Read the model definition and answer for the solid it produces. Units are mm, in the model's axes. A direction names the side the tool comes from. Round coordinates to 2 decimals unless told otherwise and drop trailing zeros. Loops run counter-clockwise (first coordinate to the right, second up) from the corner with the lowest first, then second, coordinate; pieces in that order, holes last. Notation, with made-up numbers: (34.25, -33.75) - (59.25, -33.75) arc R27 ccw to (59.25, -17.75) - close; hole circle Ø2 at (-37.75, -35). An arc over 180 degrees is marked (long way). Use one line per item in the form item = value. Start each with the question number.
Autodesk Inventor part; units mm, degrees
ref_plane "YZ Plane" through (0, 0, 0) normal (1, 0, 0) x (0, 1, 0)
ref_plane "XY Plane" through (0, 0, 0) normal (0, 0, 1) x (1, 0, 0)
sketch "Sketch1" plane through (0, 0, 0) normal (0, 1, 0) x (-1, 0, 0)
  line L0 (0, 4.5) -> (0.254, 4.5)
  line L1 (0.254, -4.5) -> (0, -4.5)
  line L2 (6.35, 4.5) -> (6.35, -4.5)
  line L3 (6.35, 7.548) -> (6.35, 4.5)
  line L4 (6.35, -7.548) -> (6.35, -4.5)
  line L5 (0.254, 4.5) -> (6.35, 7.548)
  line L6 (0.254, -4.5) -> (6.35, -7.548)
  line L7 (0, 4.5) -> (0, -4.5)
  line L8 (0, -20.9) -> (0.254, -20.9)
  line L9 (0.254, -29.9) -> (0, -29.9)
  line L10 (6.35, -20.9) -> (6.35, -29.9)
  line L11 (6.35, -17.852) -> (6.35, -20.9)
  line L12 (6.35, -32.948) -> (6.35, -29.9)
  line L13 (0.254, -20.9) -> (6.35, -17.852)
  line L14 (0.254, -29.9) -> (6.35, -32.948)
  line L15 (0, -20.9) -> (0, -29.9)
  line L16 (0, -46.3) -> (0.254, -46.3)
  line L17 (0.254, -55.3) -> (0, -55.3)
  line L18 (6.35, -46.3) -> (6.35, -55.3)
  line L19 (6.35, -43.252) -> (6.35, -46.3)
  line L20 (6.35, -58.348) -> (6.35, -55.3)
  line L21 (0.254, -46.3) -> (6.35, -43.252)
  line L22 (0.254, -55.3) -> (6.35, -58.348)
  line L23 (0, -46.3) -> (0, -55.3)
  line L24 (0, -71.7) -> (0.254, -71.7)
  line L25 (0.254, -80.7) -> (0, -80.7)
  line L26 (6.35, -71.7) -> (6.35, -80.7)
  line L27 (6.35, -68.652) -> (6.35, -71.7)
  line L28 (6.35, -83.748) -> (6.35, -80.7)
  line L29 (0.254, -71.7) -> (6.35, -68.652)
  line L30 (0.254, -80.7) -> (6.35, -83.748)
  line L31 (0, -71.7) -> (0, -80.7)
  point P0 (0, 0)
  dimension "d16" = 6.096
  dimension "d25" = 9
  dimension "d26" = 3.048
  dimension "d27" = 3.048
  dimension "d28" = 0.254
  dimension "d29" = 0.254
  dimension "d33" = 25.4
extrude "Shape" add sketch "Sketch1" along normal blind 19.05 contours L0 L5 L3 L2 L4 L6 L1 L7 | L8 L13 L11 L10 L12 L14 L9 L15 | L16 L21 L19 L18 L20 L22 L17 L23
sketch "Sketch4" plane through (0, 0, 0) normal (0, -1, 0) x (1, 0, 0)
  line L0 (0, -55.3) -> (-0.254, -55.3) construction
  line L1 (0, -46.3) -> (0, -55.3) construction
  line L2 (-6.35, -43.252) -> (-0.254, -46.3) construction
  line L3 (-6.35, -58.348) -> (-6.35, -43.252) construction
  line L4 (-0.254, -55.3) -> (-6.35, -58.348) construction
  line L5 (-0.254, -46.3) -> (0, -46.3) construction
  line L6 (0, -84.4) -> (-0.254, -84.4)
  line L7 (-0.254, -84.4) -> (-6.35, -81.352)
  line L8 (-6.35, -96.448) -> (-6.35, -81.352)
  line L9 (-0.254, -55.3) -> (-6.35, -58.348)
  line L10 (-0.254, -93.4) -> (-6.35, -96.448)
  line L11 (0, -93.4) -> (-0.254, -93.4)
  line L12 (0, -93.4) -> (0, -84.4)
  line L13 (-0.254, -46.3) -> (0, -46.3)
  line L14 (0, -46.3) -> (0, -55.3)
  point P0 (0, 0)
  dimension "d81" = 38.1
extrude "Extrusion4" add sketch "Sketch4" against normal blind 100.2792
sketch "Sketch5" plane through (0, 0, -84.4) normal (1, 0, 0) x (0, 0, -1)
  line L0 (12.048, 0) -> (12.048, 100.2792) construction
  line L1 (0, 100.2792) -> (9, 100.2792) construction
  line L2 (-91.948, 0) -> (-91.948, 19.05) construction
  line L3 (-76.852, 0) -> (-91.948, 0)
  line L4 (12.048, 0) -> (9, 0)
  line L5 (-91.948, 0) -> (12.048, 0)
  line L6 (9, 100.2792) -> (12.048, 100.2792)
  line L7 (12.048, 0) -> (12.048, 100.2792)
  line L8 (12.048, 100.2792) -> (-13.352, 100.2792)
  line L9 (-13.352, 100.2792) -> (-13.352, 19.05)
  line L10 (-29.1, 19.05) -> (-26.052, 19.05)
  line L11 (-76.852, 19.05) -> (-91.948, 19.05)
  line L12 (-13.352, 19.05) -> (-91.948, 19.05)
  line L13 (-91.948, 19.05) -> (-91.948, 0)
  point P0 (-84.4, 0)
  point P1 (-91.948, 100.2792)
  point P2 (9, 0)
  dimension "d46" = 25.4
extrude "Extrusion5" add sketch "Sketch5" along normal blind 1.27
sketch "Sketch6" plane through (-6.35, 0, -96.448) normal (-1, 0, 0) x (0, 0, 1)
  line L0 (0, 100.2792) -> (15.096, 100.2792)
  line L1 (7.548, 100.2792) -> (7.548, 0) construction
  line L2 (103.996, 0) -> (0, 0)
  circle A0 centre (7.548, 9.525) radius 1.9304
  circle A1 centre (7.548, 36.4744) radius 1.9304
  circle A2 centre (7.548, 63.4238) radius 1.9304
  circle A3 centre (7.548, 90.3732) radius 1.9304
  circle A4 centre (97.2227, 9.525) radius 1.9304
  circle A5 centre (70.2733, 9.525) radius 1.9304
  line L3 (103.996, 0) -> (103.996, 19.05)
  line L4 (25.4, 19.05) -> (103.996, 19.05) construction
  line L5 (96.448, 19.05) -> (96.448, 0) construction
  line L6 (63.5, 19.05) -> (78.596, 19.05) construction
  line L7 (71.048, 19.05) -> (71.048, 0) construction
  line L8 (63.5, 0) -> (78.596, 0) construction
  line L9 (63.5, 0) -> (63.5, 19.05)
  line L10 (78.596, 0) -> (78.596, 19.05)
  dimension "d54" = 26.9494
  dimension "d48" = 3.8608
  dimension "d51" = 26.9494
  dimension "d57" = 3.8608
  dimension "d60" = 26.9494
  dimension "d69" = 0.7747
hole "Hole1" at (-6.35, 90.3732, -88.9) at (-6.35, 63.4238, -88.9) at (-6.35, 36.4744, -88.9) at (-6.35, 9.525, -88.9) at (-6.35, 9.525, -26.1747) at (-6.35, 9.525, 0.7747) direction (1, 0, 0) diameter 3.8608 end through all counterbore diameter 8.89 counterbore depth 3.2512
ref_plane "Work Plane1" through (0, 9.525, 0) normal (0, 1, 0) x (-1, 0, 0)
ref_plane "Work Plane2" through (8.746, 0, -88.9) normal (0, 0, -1) x (0, 1, 0)
equation "\"d27\" = d26"
equation "\"d29\" = d28"
properties part number "Lift mount insert left"
1) For faces 3 (the flat face through (-3.259, 9.392, -19.397)), 4 (the flat face through (-3.259, 49.438, -94.903)), 5 (the flat face through (-3.099, 10.5, -87)), determine the directions among +Z, -Z, +X, -X, +Y, -Y from which every point of the face is accessible in a straight line to the end or side of a thin tool.
2) Straight lines are drawn through the part: line 1 (Y direction, x = -3.25, z = -89); line 2 (Y direction, x = -1.5, z = -88.9); line 3 (X direction, y = 8, z = -71). For each, find the intervals that lie inside material, in ascending order. Write a range as from..to.
3) A cutting plane is placed at C-C on z = -88.9. Count the separate pieces of the cut face and the enclosed holes in it, plus the area to 3 significant figures.
4) A cutting plane is placed at A-A on z = -26.5. Write down the section's boundary in (x, y).
5) Determine the mould class of faces 1 (the flat face through (-3.259, 9.392, -6.003)), 2 (the cylindrical face through (-0.884, 8.945, -87.059)) for opening direction Y: +Y half, -Y half, draft (parallel to the pull), parting line (faces both ways), or undercut.
6) Flat-ended cylindrical pins translate along their axes: pin 1 (10 mm diameter, centred on y = 20, z = -55.5, fed in from +X); pin 2 (1 mm diameter, centred on x = -1.5, y = 36.5, fed in from -Z); pin 3 (4 mm diameter, centred on x = -3.5, y = 75, fed in from -Z); pin 4 (4 mm diameter, centred on x = -4.5, z = -52.5, fed in from +Y). Find the tip coordinate at first contact, or state that the pin passes through.
7) A cutting plane is placed at D-D on z = -41. Write down the section's boundary in (x, y), plus the area to 3 significant figures.
8) A cutting plane is placed at B-B on y = 76. Write down the section's boundary in (x, z), plus the area to 3 significant figures.
Checks:
q1.face_3 = +Y, -Y
q1.face_4 = -Z, +Y, -Y
q1.face_5 = -X
q2.line_1 = 0..5.08, 13.97..32.03, 40.92..58.98, 67.87..85.93, 94.82..100.28
q2.line_2 = 0..7.59, 11.46..34.54, 38.4..61.49, 65.35..88.44, 92.3..100.28
q2.line_3 = 0..1.27
q3.separate_pieces = 5
q3.enclosed_holes = 0
q3.area = 581 mm²
q4.outline = (-6.35, 0) - (1.27, 0) - (1.27, 7.62) - (-3.1, 7.62) - (-3.1, 5.09) - (-6.35, 5.09) - close; (-6.35, 13.96) - (-3.1, 13.96) - (-3.1, 11.43) - (1.27, 11.43) - (1.27, 19.05) - (-6.35, 19.05) - close
q5.face_1 = draft
q5.face_2 = undercut
q6.pin_1 = 1.27
q6.pin_2 = -94.27
q6.pin_3 = -96.02
q6.pin_4 = 19.05
q7.outline = (0, 0) - (1.27, 0) - (1.27, 19.05) - (0, 19.05) - close
q7.area = 24.2 mm²
q8.outline = (-6.35, -96.45) - (-0.25, -93.4) - (0, -93.4) - (0, -96.45) - (1.27, -96.45) - (1.27, -71.05) - (0, -71.05) - (0, -84.4) - (-0.25, -84.4) - (-6.35, -81.35) - close
q8.area = 108 mm²
